```python
from build123d import *

# Parameters (mm, degrees)
SKETCH1_W                        = 5.334
SKETCH1_H                        = 19.05
F_1_4_0_25_DIAMETER_HOLE1_D      = 6.35
F_21_0_159_DIAMETER_HOLE1_REACH  = 21.654
F_21_0_159_DIAMETER_HOLE1_BORE_R = 2.0193


with BuildPart() as part:
    # Sketch1 → Revolve1 (revolve)
    with BuildSketch(Plane.XY, mode=Mode.PRIVATE) as revolve1_sk:
        with Locations((2.667, 9.525)):
            Rectangle(SKETCH1_W, SKETCH1_H)
    revolve(revolve1_sk.sketch.rotate(Axis((0, 19.05, 0), (0, -1, 0)), 270), axis=Axis((0, 19.05, 0), (0, -1, 0)))

    # 1/4 (0.25) Diameter Hole1 (through all)
    with Locations(Plane(origin=(0, 0, 0), x_dir=(-1, 0, 0), z_dir=(0, -1, 0))):
        with Locations((0, 0)):
            Hole(F_1_4_0_25_DIAMETER_HOLE1_D / 2)

    # #21 (0.159) Diameter Hole1 bore (on position points) → #21 (0.159) Diameter Hole1 (cut, up to next)
    with BuildSketch(Plane(origin=(0, 3.429, 5.334), x_dir=(1, 0, 0), z_dir=(0, 0, 1)), mode=Mode.PRIVATE) as f_21_0_159_diameter_hole1_sk1:
        Circle(F_21_0_159_DIAMETER_HOLE1_BORE_R)
    f_21_0_159_diameter_hole1_tool1 = extrude(f_21_0_159_diameter_hole1_sk1.sketch, amount=-F_21_0_159_DIAMETER_HOLE1_REACH, mode=Mode.PRIVATE) & part.part
    add(f_21_0_159_diameter_hole1_tool1.solids().sort_by_distance((0, 3.429, 5.334))[0], mode=Mode.SUBTRACT)


solid = part.part
```
Can you work these out from the model? Positions are in its coordinate system, mm. A direction names the side the tool comes from. Give positions to 0.01 mm unless a question says otherwise; leave off trailing zeros. Loops run counter-clockwise (first coordinate to the right, second up) from the corner with the lowest first, then second, coordinate; pieces in that order, holes last. Notation, with made-up numbers: M 15.5,-0.5 L 28.5,-0.5 A22 ccw 28.5,32.5 Z; hole C 86.25,-34.75 d2. An arc over 180 degrees is marked long. Use one line per item in the form item = value. Start each with the question number.
(1) I'm going to push flat-ended pins straight in: P1, Ø2, axis at x = -2.5, y = 6, coming from the +Z side; P2, Ø5, axis at x = -2.5, y = 7.5, coming from the +Z side; P3, Ø1, axis at x = 2.5, y = 12, coming from the -Z side; P4, Ø3.5, axis at x = 0, y = 3.429, coming from the +Z side. Where does each tip first touch, or does it pass through?
(2) I want a section at A-A, the plane z = 0. Write out the boundary of the cut face in (x, y) (3 decimals), and give its area (3 significant figures).
(3) I want a section at D-D, the plane z = 1.25. Write out the boundary of the cut face in (x, y), and give its area (3 significant figures).
(4) On a 3-axis mill with a long thin cutter (end or side, diameter ignored), from which of +Z, -Z, +X, -X, +Y, -Y can I reach the whole of each face in a straight line? I mean faces 4 (the cylindrical face through (1.926, 4.036, 3.912)), 5 (the flat face through (-3.5, 19.05, -0.1)). Say none if no direction works.
(5) Thinking about a two-plate mould opening in X: for faces 1 (the cylindrical face through (-0.41, 9.66, -3.15)), 2 (the cylindrical face through (-2.04, 9.66, -4.93)), 3 (the flat face through (-3.5, 0, -0.1)), which applies, released by +X, released by -X, zero draft, split by the parting line, or undercut?
(6) I want a section at C-C, the plane y = 6.5. Write out the boundary of the cut face in (x, z) (3 decimals), and give its area (3 significant figures).
(7) I want a section at B-B, the plane x = 0. Write out the boundary of the cut face in (y, z) (3 decimals), and give its area (3 significant figures).
(8) Please list where these lines run through material, in increasing order: line 1 (Y direction, x = 0, z = 4.4); line 2 (Z direction, x = 0, y = 15.5) (3 decimals); line 3 (X direction, y = 5.25, z = 0.75).
Worked out:
q1.P1 = 5.12
q1.P2 = 5.33
q1.P3 = -4.94
q1.P4 = -2.65
q2.outline = M -5.334,0 L -3.175,0 L -3.175,19.05 L -5.334,19.05 Z; M 3.175,0 L 5.334,0 L 5.334,19.05 L 3.175,19.05 Z
q2.area = 82.3 mm²
q3.outline = M -5.19,0 L -2.92,0 L -2.92,19.05 L -5.19,19.05 Z; M 2.92,0 L 5.19,0 L 5.19,19.05 L 2.92,19.05 Z
q3.area = 86.4 mm²
q4.face_4 = +Z
q4.face_5 = +Z, -Z, +X, -X, +Y
q5.face_1 = undercut
q5.face_2 = split by the parting line
q5.face_3 = zero draft
q6.outline = C 0,0 d10.668; hole C 0,0 d6.35
q6.area = 57.7 mm²
q7.outline = M 0,-5.334 L 19.05,-5.334 L 19.05,-3.175 L 0,-3.175 Z; M 0,3.175 L 1.41,3.175 L 1.41,5.334 L 0,5.334 Z; M 5.448,3.175 L 19.05,3.175 L 19.05,5.334 L 5.448,5.334 Z
q7.area = 73.5 mm²
q8.line_1 = 0 to 1.41, 5.45 to 19.05
q8.line_2 = -5.334 to -3.175, 3.175 to 5.334
q8.line_3 = -5.28 to -3.09, 3.09 to 5.28
